```python
from build123d import *

# Parameters (mm, degrees)
BOSS_EXTRUDE1_DEPTH = 19.05
CUT_EXTRUDE1_REACH  = 118.056
SKETCH2_R           = 6.35
CUT_EXTRUDE2_REACH  = 121.753
SKETCH3_R           = 4.765


with BuildPart() as part:
    # Sketch1 → Boss-Extrude1 (new, symmetric)
    with BuildSketch(Plane.XY):
        with BuildLine():
            Line((0, 0), (53.98, 0))
            ThreePointArc((53.98, 0), (60.718727625, -2.791272375), (63.51, -9.53))
            Line((63.51, -9.53), (63.51, -85.72))
            ThreePointArc((63.51, -85.72), (60.718727625, -92.458727625), (53.98, -95.25))
            Line((53.98, -95.25), (9.39, -95.25))
            Line((9.39, -95.25), (-25.15094394, -66.266706679))
            Line((-25.15094394, -66.266706679), (-20.953540849, -61.264436466))
            Line((-20.953540849, -61.264436466), (11.76672563, -88.72))
            Line((11.76672563, -88.72), (53.98, -88.72))
            ThreePointArc((53.98, -88.72), (56.101320344, -87.841320344), (56.98, -85.72))
            Line((56.98, -85.72), (56.98, -9.53))
            ThreePointArc((56.98, -9.53), (56.101320344, -7.408679656), (53.98, -6.53))
            Line((53.98, -6.53), (0, -6.53))
            Line((0, -6.53), (0, 0))
        make_face()
    extrude(amount=BOSS_EXTRUDE1_DEPTH, both=True)

    # Sketch2 → Cut-Extrude1 (cut, up to next)
    with BuildSketch(Plane(origin=(0, 0, 0), x_dir=(1, 0, 0), z_dir=(0, 1, 0)), mode=Mode.PRIVATE) as cut_extrude1_sk1:
        with Locations(Location((19.04, 0, 0), (0, 0, 270))):
            Circle(SKETCH2_R)
    cut_extrude1_tool1 = extrude(cut_extrude1_sk1.sketch, amount=-CUT_EXTRUDE1_REACH, mode=Mode.PRIVATE) & part.part
    add(cut_extrude1_tool1.solids().sort_by_distance((19.04, 0, 0))[0], mode=Mode.SUBTRACT)

    # Sketch3 → Cut-Extrude2 (cut, up to next)
    with BuildSketch(Plane(origin=(-43.021747431, -51.271322061, 0), x_dir=(0.7660444431189771, -0.6427876096865404, 0), z_dir=(-0.6427876096865404, -0.7660444431189771, 0)), mode=Mode.PRIVATE) as cut_extrude2_sk1:
        with Locations((44.138677144, 0)):
            Circle(SKETCH3_R)
    cut_extrude2_tool1 = extrude(cut_extrude2_sk1.sketch, amount=-CUT_EXTRUDE2_REACH, mode=Mode.PRIVATE) & part.part
    add(cut_extrude2_tool1.solids().sort_by_distance((-9.209559, -79.643117, 0))[0], mode=Mode.SUBTRACT)


solid = part.part
```
Read the model definition and answer for the solid it produces. Units are mm, in the model's axes. A direction names the side the tool comes from. Coordinates: 2 decimals unless noted, no trailing zeros. Write each loop counter-clockwise with the first axis right and the second up, starting at its lowest first coordinate (ties: lowest second). Pieces come first, ordered by that corner, then holes. Notation, with made-up numbers: (-37.75, 9) -> (6.25, 9) arc R15 cw to (6.25, 34) -> close; hole circle Ø10 at (67, -29.5). An arc over 180 degrees is marked (long way). Write item = value, one per line.
(1) Which of the six approach directions +Z, -Z, +X, -X, +Y, -Y give full straight-line access (tool end or side, diameter ignored) to faces 5 (the face through (59, -47, -19.05)), 6 (the face through (56.08, -87.86, 0.27)), 7 (the face through (0, -3, 0)), 8 (the face through (56.12, -7.43, 0.27)), 9 (the face through (25.336, -3.219, -0.827))?
From the geometry:
face_5 = -Z, +X, -X, +Y, -Y
face_6 = +Z, -Z
face_7 = +Z, -Z, -X, +Y
face_8 = +Z, -Z, -X
face_9 = +Y
(2) Section C-C on z = 0 is taken. Write down the section's boundary in (x, y), plus the area to 3 significant figures.
From the geometry:
outline = (-25.15, -66.27) -> (-12.86, -76.58) -> (-8.66, -71.58) -> (-20.95, -61.26) -> close; (-5.56, -82.71) -> (9.39, -95.25) -> (53.98, -95.25) arc R9.53 ccw to (63.51, -85.72) -> (63.51, -9.53) arc R9.53 ccw to (53.98, 0) -> (25.39, 0) -> (25.39, -6.53) -> (53.98, -6.53) arc R3 cw to (56.98, -9.53) -> (56.98, -85.72) arc R3 cw to (53.98, -88.72) -> (11.77, -88.72) -> (-1.36, -77.7) -> close; (0, -6.53) -> (12.69, -6.53) -> (12.69, 0) -> (0, 0) -> close
area = 1,400 mm2
(3) For a pull along Y with two mould halves and no side action, classify faces 1 (the face through (63.51, -47, 0)), 2 (the face through (-23.08, -63.8, 0.27)), 3 (the face through (-1.19, -77.85, 0.27)), 4 (the face through (60.792, -92.384, 0.267)) as +Y half, -Y half, draft (parallel to the pull), parting line (faces both ways), or undercut.
From the geometry:
face_1 = draft
face_2 = +Y half
face_3 = undercut
face_4 = -Y half
(4) Straight lines are drawn through the part: L1, parallel to Y at x = 39.5, z = -4; L2, parallel to X at y = -14.5, z = -17; L3, parallel to Y at x = 5, z = -6.5. For each, find the intervals that lie inside material, in ascending order. Write a range as from..to.
From the geometry:
L1 = -95.25..-88.72, -6.53..0
L2 = 56.98..63.51
L3 = -91.57..-83.04, -6.53..0
(5) Section D-D on y = -34 is taken. Write down the section's boundary in (x, z).
From the geometry:
outline = (56.98, -19.05) -> (63.51, -19.05) -> (63.51, 19.05) -> (56.98, 19.05) -> close
(6) Section B-B on z = -12 is taken. Write down the section's boundary in (x, y), plus the area to 3 significant figures.
From the geometry:
outline = (-25.15, -66.27) -> (9.39, -95.25) -> (53.98, -95.25) arc R9.53 ccw to (63.51, -85.72) -> (63.51, -9.53) arc R9.53 ccw to (53.98, 0) -> (0, 0) -> (0, -6.53) -> (53.98, -6.53) arc R3 cw to (56.98, -9.53) -> (56.98, -85.72) arc R3 cw to (53.98, -88.72) -> (11.77, -88.72) -> (-20.95, -61.26) -> close
area = 1,550 mm2
(7) Section A-A on x = 19.04 is taken. Write down the section's boundary in (y, z), plus the area to 3 significant figures.
From the geometry:
outline = (-95.25, -19.05) -> (-88.72, -19.05) -> (-88.72, 19.05) -> (-95.25, 19.05) -> close; (-6.53, -19.05) -> (0, -19.05) -> (0, -6.35) -> (-6.53, -6.35) -> close; (-6.53, 6.35) -> (0, 6.35) -> (0, 19.05) -> (-6.53, 19.05) -> close
area = 415 mm2
(8) Given pin 1 Ø3 at (y, z) = (-68, -0.5) entering from -X; pin 2 Ø10 at (x, y) = (14.5, -15.5) entering from +Z; pin 3 Ø3 at (y, z) = (-48.5, -8) entering from -X; pin 4 Ø1.5 at (y, z) = (-77.5, -5.5) entering from -X, each flat-ended and moving along its own axis, determine where each tip first touches the part or whether it passes through.
From the geometry:
pin_1 = -24.87
pin_2 = through
pin_3 = 56.98
pin_4 = -12.66
